```python
from build123d import *

# Parameters (mm, degrees)
SKETCH1_W           = 14
SKETCH1_H           = 14
SKETCH1_R           = 2
BOSS_EXTRUDE1_DEPTH = 10
SKETCH3_W           = 4
SKETCH3_H           = 18
SKETCH3_W_2         = 12
SKETCH3_H_2         = 14
CUT_EXTRUDE1_DEPTH  = 7
FILLET1_R           = 4
FILLET2_R           = 2
SKETCH4_W           = 2
SKETCH4_H           = 9
BOSS_EXTRUDE2_DEPTH = 4
FILLET3_R           = 2


with BuildPart() as part:
    # Sketch1 → Boss-Extrude1 (new body)
    # profile 1 of 2: a face of its own
    with BuildSketch(Plane(origin=(0, 0, 0), x_dir=(1, 0, 0), z_dir=(0, 1, 0))):
        Polygon((14, 14), (14, 0), (14, -4.5), (24, -4.5), (24, 0), (17, 0), (17, 14), (24, 14), (24, 18.5), (14, 18.5), align=None)
    # profile 2 of 2: a face of its own
    with BuildSketch(Plane(origin=(0, 0, 0), x_dir=(1, 0, 0), z_dir=(0, 1, 0))):
        with Locations((7, 7)):
            Rectangle(SKETCH1_W, SKETCH1_H)
        with Locations(Location((4, 7, 0), (0, 0, 270))):
            Circle(SKETCH1_R, mode=Mode.SUBTRACT)
    extrude(amount=BOSS_EXTRUDE1_DEPTH)

    # Sketch3 → Cut-Extrude1 (cut)
    with BuildSketch(Plane(origin=(0, 10, 0), x_dir=(1, 0, 0), z_dir=(0, 1, 0))):
        with Locations((19, 7)):
            Rectangle(SKETCH3_W, SKETCH3_H)
        with Locations((6, 7)):
            Rectangle(SKETCH3_W_2, SKETCH3_H_2)
    extrude(amount=-CUT_EXTRUDE1_DEPTH, mode=Mode.SUBTRACT)

    # Fillet1
    fillet1_edges = [part.edges().sort_by_distance(p)[0] for p in [
        (12, 3, -7),
    ]]
    fillet(fillet1_edges, radius=FILLET1_R)

    # Fillet2
    fillet2_edges = [part.edges().sort_by_distance(p)[0] for p in [
        (12, 10, -7),
    ]]
    fillet(fillet2_edges, radius=FILLET2_R)

    # Sketch4 → Boss-Extrude2 (add)
    with BuildSketch(Plane.XZ):
        with Locations((8.05, -7)):
            Rectangle(SKETCH4_W, SKETCH4_H)
    extrude(amount=BOSS_EXTRUDE2_DEPTH)

    # Fillet3
    fillet3_edges = [part.edges().sort_by_distance(p)[0] for p in [
        (9.05, 0, -7),
    ]]
    fillet(fillet3_edges, radius=FILLET3_R)


solid = part.part
```
Geometry: final body of the model. Coordinates: model frame, mm. A direction names the side the tool comes from. Give positions to 0.01 mm unless a question says otherwise; leave off trailing zeros. Loops run counter-clockwise (first coordinate to the right, second up) from the corner with the lowest first, then second, coordinate; pieces in that order, holes last. Notation, with made-up numbers: (30.5, 58.25) -> (58.5, 58.25) arc R10 cw to (58.5, 76.25) -> close; hole circle Ø8 at (-32, 26). An arc over 180 degrees is marked (long way). Return JSON: item names as keys, results as strings.
Item 1: Section B-B, the plane z = -7. Output: boundary loops of the cut face in (x, y), plus the area to 3 significant figures.
Filled in:
{"outline": "(0, 0) -> (2, 0) -> (2, 3) -> (0, 3) -> close; (6, 0) -> (7.05, 0) -> (7.05, -4) -> (9.05, -4) -> (9.05, -2) arc R2 cw to (11.05, 0) -> (17, 0) -> (17, 10) -> (14, 10) arc R2 ccw to (12, 8) -> (12, 7) arc R4 cw to (8, 3) -> (6, 3) -> close", "area": "85.4 mm^2"}
Item 2: Pin query (flat end, axial travel): P1, Ø8, axis at x = 3.5, z = -6.5, coming from the -Y side; P2, Ø4.5, axis at x = 9, y = -2, coming from the -Z side; P3, Ø1, axis at x = 19, z = -15, coming from the +Y side; P4, Ø3, axis at x = 6, y = 3.5, coming from the +Z side. Return the tip coordinate at first contact, or that it passes through.
Filled in:
{"P1": "y = -4", "P2": "z = -14", "P3": "y = 3", "P4": "z = 0"}
Item 3: Mould query, pull axis Z, two halves, no side actions, for faces 1 (the flat face through (17, 5, -7)), 2 (the flat face through (8, -2, -11.5)), 3 (the flat face through (9.05, -3, -7)), 4 (the flat face through (21.3, 3.8, 0)). Classes: released by +Z, released by -Z, zero draft, split by the parting line, or undercut.
Filled in:
{"face 1": "undercut", "face 2": "released by -Z", "face 3": "zero draft", "face 4": "undercut"}
Item 4: Access query for faces 5 (the flat face through (14, 5, 2)), 6 (the flat face through (19, 7, -16)), 7 (the flat face through (8, -2, -2.5)). Directions: +Z, -Z, +X, -X, +Y, -Y. A direction counts if a zero-diameter tool reaches every point of the face in a straight line with its end or side. Return the directions, or none.
Filled in:
{"face 5": "+Z, -X, +Y, -Y", "face 6": "+Y", "face 7": "+Z, +X, -X, -Y"}
Item 5: Section C-C, the plane y = 7.5. Output: boundary loops of the cut face in (x, z).
Filled in:
{"outline": "(12, -14) -> (14, -14) -> (14, -18.5) -> (24, -18.5) -> (24, -14) -> (21, -14) -> (21, -16) -> (17, -16) -> (17, 2) -> (21, 2) -> (21, 0) -> (24, 0) -> (24, 4.5) -> (14, 4.5) -> (14, 0) -> (12, 0) -> close"}
Item 6: Section A-A, the plane x = 18.75. Output: boundary loops of the cut face in (y, z), plus the area to 3 significant figures.
Filled in:
{"outline": "(0, -18.5) -> (10, -18.5) -> (10, -16) -> (3, -16) -> (3, -14) -> (0, -14) -> close; (0, 0) -> (3, 0) -> (3, 2) -> (10, 2) -> (10, 4.5) -> (0, 4.5) -> close", "area": "62.0 mm^2"}
Item 7: Section D-D, the plane z = 1.5. Output: boundary loops of the cut face in (x, y).
Filled in:
{"outline": "(14, 0) -> (24, 0) -> (24, 10) -> (21, 10) -> (21, 3) -> (17, 3) -> (17, 10) -> (14, 10) -> close"}
Item 8: Line query: line 1 (X direction, y = 1.2, z = -7); line 2 (Z direction, x = 4, y = 1.35); line 3 (Z direction, x = 22.75, y = 9). Output: solid intervals per line, ascending.
Filled in:
{"line 1": "0 to 2, 6 to 17", "line 2": "-14 to -9, -5 to 0", "line 3": "-18.5 to -14, 0 to 4.5"}
